Source: three-view drawing plus pictorial views. Frame: mm from the lowest corner of the part. A direction names the side the tool comes from. Give positions to 0.01 mm unless a question says otherwise; leave off trailing zeros. Loops run counter-clockwise (first coordinate to the right, second up) from the corner with the lowest first, then second, coordinate; pieces in that order, holes last. Notation, with made-up numbers: M 47.5,-14 L 93.5,-14 A13 cw 93.5,3 Z; hole C -18.75,-10.75 d3. An arc over 180 degrees is marked long. One line per item, written item: value. Start each with the question number.
(1) Access query for the marked faces 1 and 2. Directions: +Z, -Z, +X, -X, +Y, -Y. A direction counts if a zero-diameter tool reaches every point of the face in a straight line with its end or side. Return the directions, or none.
(2) Section D-D on y = 4.5. Output: boundary loops of the cut face in (x, z), plus the area to 3 significant figures.
(3) Section C-C on z = 9. Output: boundary loops of the cut face in (x, y), plus the area to 3 significant figures.
(4) Pin query (flat end, axial travel): P1, Ø3, axis at x = 10.5, z = 2.5, coming from the +Y side; P2, Ø8, axis at y = 21.5, z = 7, coming from the -X side; P3, Ø6, axis at x = 24, z = 10.5, coming from the -Y side. Return the tip coordinate at first contact, or that it passes through.
(5) Ray query, line 1 along Y through (x, z) = (17, 6); line 2 along Y through (x, z) = (16.5, 11.75) (1 decimal); line 3 along Z through (x, y) = (17, 7). Return the intervals inside material, ascending. Write a range as from..to.
(6) Section A-A on y = 17. Output: boundary loops of the cut face in (x, z), plus the area to 3 significant figures.
(7) Section B-B on x = 25. Output: boundary loops of the cut face in (y, z), plus the area to 3 significant figures.
(8) Pull-direction query (Y, two-part tool) for the marked faces 3, 4 and 5; classes: released by +Y, released by -Y, zero draft, split by the parting line, or undercut.
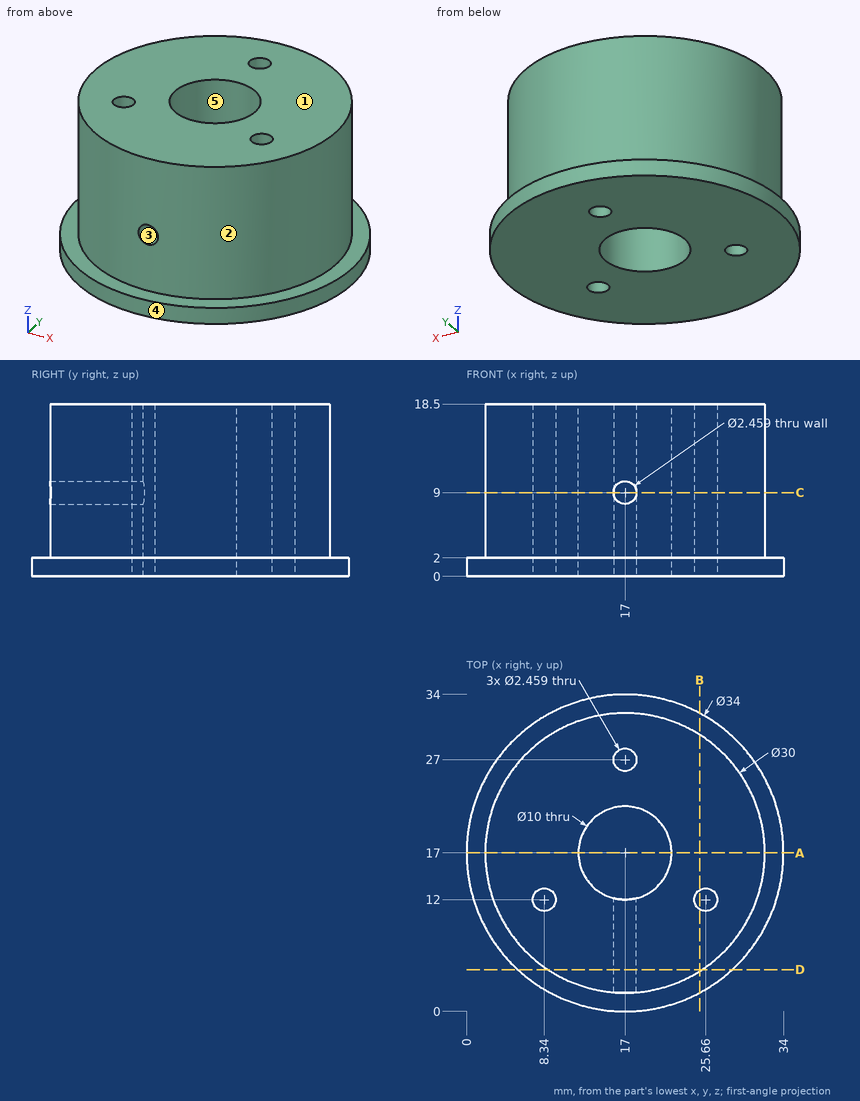
Output values:
1. face 1: +Z, +X, -X, +Y, -Y
1. face 2: +Z
2. outline: M 5.48,0 L 28.52,0 L 28.52,2 L 25.29,2 L 25.29,18.5 L 8.71,18.5 L 8.71,2 L 5.48,2 Z; hole C 17,9 d2.46
2. area: 315 mm²
3. outline: M 15.77,2.05 L 15.77,12.15 A5 cw long 18.23,12.15 L 18.23,2.05 A15 ccw long Z; hole C 8.34,12 d2.46; hole C 17,27 d2.46; hole C 25.66,12 d2.46
3. area: 589 mm²
4. P1: stops at y = 33.22
4. P2: stops at x = 2.01
4. P3: stops at y = 2.54
5. line 1: y = 2..12, 22..25.77, 28.23..32
5. line 2: y = 2..12, 22..25.9, 28.1..32
5. line 3: z = 0..7.77, 10.23..18.5
6. outline: M 0,0 L 12,0 L 12,18.5 L 2,18.5 L 2,2 L 0,2 Z; M 22,0 L 34,0 L 34,2 L 32,2 L 32,18.5 L 22,18.5 Z
6. area: 378 mm²
7. outline: M 2,0 L 10.96,0 L 10.96,18.5 L 4.31,18.5 L 4.31,2 L 2,2 Z; M 13.04,0 L 32,0 L 32,2 L 29.69,2 L 29.69,18.5 L 13.04,18.5 Z
7. area: 440 mm²
8. face 3: zero draft
8. face 4: split by the parting line
8. face 5: undercut
